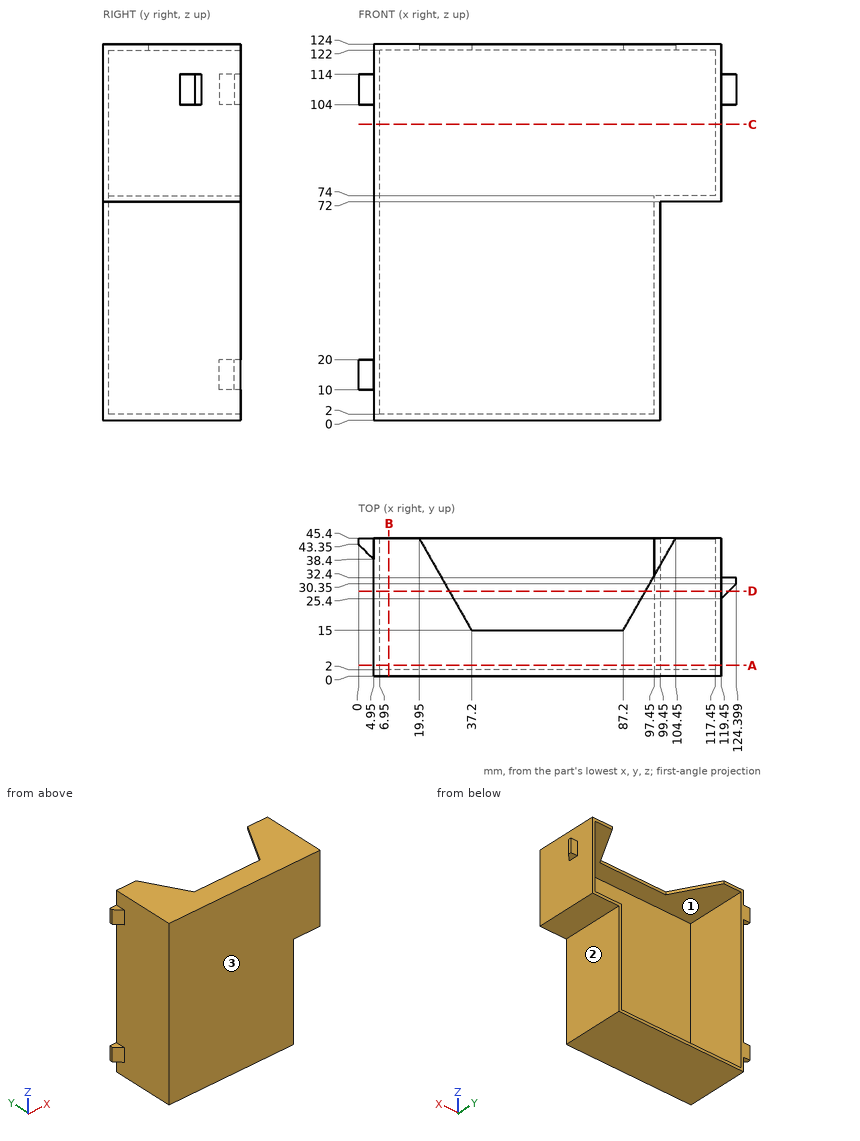
Geometry: see drawing. Coordinates: mm, zero at the bounding-box minimum. A direction names the side the tool comes from. Round coordinates to 2 decimals unless told otherwise and drop trailing zeros. Loops run counter-clockwise (first coordinate to the right, second up) from the corner with the lowest first, then second, coordinate; pieces in that order, holes last. Notation, with made-up numbers: (23, 82) - (61, 82) arc R14 cw to (61, 100) - close; hole circle Ø3 at (47, -4). An arc over 180 degrees is marked (long way). Use CSV: the item, a comma, the result in double quotes.
Q1. Section query C-C, the plane z = 97.5. Output: boundary loops of the cut face in (x, y).
Reported:
outline,"(4.95, 0) - (119.45, 0) - (119.45, 45.4) - (117.45, 45.4) - (117.45, 2) - (6.95, 2) - (6.95, 45.4) - (4.95, 45.4) - close"
Q2. Section query A-A, the plane y = 3.5. Output: boundary loops of the cut face in (x, z).
Reported:
outline,"(4.95, 0) - (99.45, 0) - (99.45, 72) - (119.45, 72) - (119.45, 124) - (4.95, 124) - close; hole (6.95, 2) - (97.45, 2) - (97.45, 74) - (117.45, 74) - (117.45, 122) - (6.95, 122) - close"
Q3. Pin query (flat end, axial travel): pin 1 Ø21.5 at (y, z) = (16.5, 62.5) entering from +X; pin 2 Ø16 at (x, y) = (104.5, 27) entering from -Z; pin 3 Ø3 at (y, z) = (8.5, 39.5) entering from +X; pin 4 Ø8 at (x, z) = (28.5, 32) entering from +Y. Return the tip coordinate at first contact, or that it passes through.
Reported:
pin 1,"x = 119.45"
pin 2,"z = 0"
pin 3,"x = 99.45"
pin 4,"y = 2"
Q4. Ray query, line 1 along X through (y, z) = (4.5, 67); line 2 along Z through (x, y) = (58, 14.5); line 3 along X through (y, z) = (35, 110.5). Return the intervals inside material, ascending.
Reported:
line 1,"4.95 to 6.95, 97.45 to 99.45"
line 2,"0 to 2, 122 to 124"
line 3,"4.95 to 6.95, 117.45 to 119.45"
Q5. Section query D-D, the plane y = 28. Output: boundary loops of the cut face in (x, z).
Reported:
outline,"(4.95, 0) - (99.45, 0) - (99.45, 72) - (119.45, 72) - (119.45, 104) - (122.05, 104) - (122.05, 114) - (119.45, 114) - (119.45, 124) - (94.58, 124) - (94.58, 122) - (117.45, 122) - (117.45, 74) - (97.45, 74) - (97.45, 2) - (6.95, 2) - (6.95, 122) - (29.82, 122) - (29.82, 124) - (4.95, 124) - close"
Q6. Section query B-B, the plane x = 10. Output: boundary loops of the cut face in (y, z).
Reported:
outline,"(0, 0) - (45.4, 0) - (45.4, 2) - (2, 2) - (2, 122) - (45.4, 122) - (45.4, 124) - (0, 124) - close"
Q7. Reachability of the marked faces 1, 2 and 3 from +Z, -Z, +X, -X, +Y, -Y: full face, straight path, thin tool, end or side. Return the list, or none.
Reported:
face 1,"+Y"
face 2,"-Z, +X, +Y, -Y"
face 3,"+Z, -Z, +X, -X, -Y"
